from build123d import *

# Parameters (mm, degrees)
F1_DEPTH = 76.2
F0_R     = 3.17989
F2_DEPTH = 12.7
F0_R_2   = 3.190914
F3_DEPTH = 12.7
F0_W     = 38.1
F0_H     = 50.8
F4_DEPTH = 12.7


with BuildPart() as f1:
    # F0 (on Top) → F1 (new body)
    with BuildSketch(Plane.XY):
        Polygon((-63.963963, 7.02602), (-70.885196, 7.02602), (-70.885196, 6.905661), (-70.885196, -29.80398), (-20.085196, -29.80398), (-20.085196, 6.905661), (-20.085196, 7.02602), (-25.863963, 7.02602), align=None)
    extrude(amount=F1_DEPTH)

    # F0 (on Top) → F2 (join)
    with BuildSketch(Plane.XY):
        Polygon((-70.885196, -29.80398), (-70.885196, 6.905661), (-108.985196, 6.905661), (-108.985196, -29.924339), (-70.885196, -29.924339), align=None)
        with Locations((-89.978054, -11.557001)):
            Circle(F0_R, mode=Mode.SUBTRACT)
    extrude(amount=F2_DEPTH)

    # F0 (on Top) → F3 (join)
    with BuildSketch(Plane.XY):
        Polygon((-20.085196, 6.905661), (-20.085196, -29.80398), (-20.085196, -29.924339), (18.014804, -29.924339), (18.014804, 6.905661), align=None)
        with Locations((-0.353005, -11.161889)):
            Circle(F0_R_2, mode=Mode.SUBTRACT)
    extrude(amount=F3_DEPTH)

    # F0 (on Top) → F4 (join)
    with BuildSketch(Plane.XY):
        with Locations((-44.913963, 32.42602)):
            Rectangle(F0_W, F0_H)
        with Locations((-55.91448, 45.011953)):
            Circle(F0_R, mode=Mode.SUBTRACT)
        with Locations((-44.610804, 32.42602)):
            Circle(F0_R, mode=Mode.SUBTRACT)
        with Locations((-34.018744, 45.011953)):
            Circle(F0_R, mode=Mode.SUBTRACT)
    extrude(amount=F4_DEPTH)


solid = f1.part
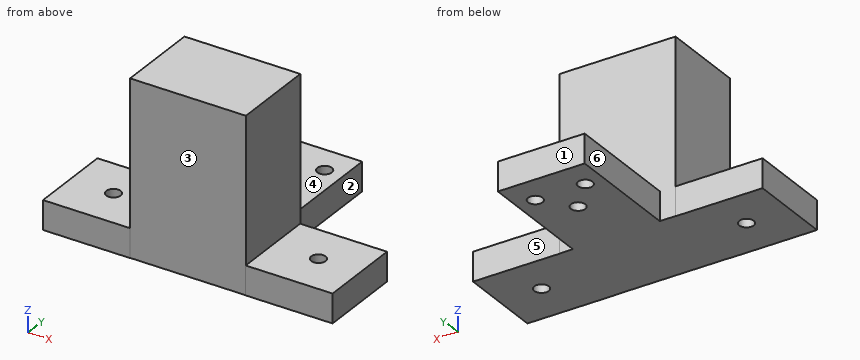
Geometry check sheet. Reference: the model listing, model coordinates, mm. Face numbers are marked on the shaded views. A direction names the side the tool comes from. Give positions to 0.01 mm unless a question says otherwise; leave off trailing zeros. Order: outer loops, then holes, each group sorted by start corner. A loop starts at its lowest first (then second) coordinate and runs counter-clockwise, first axis right, second up.
1) Material ranges on probe 1 along Z at (x, y) = (-1, 6); probe 2 along X at (y, z) = (-16.5, 29); probe 3 along Y at (x, z) = (-63.5, 60.5), recorded low to high.
Results are:
probe 1: z = 0 to 12.7
probe 2: x = -70.89 to -20.09
probe 3: y = -29.8 to 7.03
2) Cross-section at A-A (y = -6). Record the boundary of the cut face in (x, z), then the cut area to 3 significant figures.
Results are:
outline: (-108.99, 0) - (18.01, 0) - (18.01, 12.7) - (-20.09, 12.7) - (-20.09, 76.2) - (-70.89, 76.2) - (-70.89, 12.7) - (-108.99, 12.7) - close
area: 4,840 mm2
3) Gauge pin test, flat ends, axial feed: pin 1 (14 mm diameter, centred on x = 6, z = 9.5, fed in from +Y); pin 2 (10 mm diameter, centred on y = 36.5, z = 3.5, fed in from -X); pin 3 (11.5 mm diameter, centred on x = -40.5, y = 33, fed in from +Z). Record the tip position at first contact, or that the pin passes through.
Results are:
pin 1: stops at y = 6.91
pin 2: stops at x = -63.96
pin 3: stops at z = 12.7
4) Tool access check on the marked faces 4, 5 and 6. Record the directions out of +Z, -Z, +X, -X, +Y, -Y that give a thin tool (end or side, any length) a straight path to the whole face; none if there is none.
Results are:
face 4: +Z, +X, -X, +Y
face 5: +Z, -Z, +X, +Y
face 6: +Z, -Z, -X, +Y
5) Cross-section at C-C (x = -67.5). Record the boundary of the cut face in (y, z), then the cut area to 3 significant figures.
Results are:
outline: (-29.8, 0) - (7.03, 0) - (7.03, 76.2) - (-29.8, 76.2) - close
area: 2,810 mm2
6) Draft check along X on the marked faces 1, 2 and 3. Enter one of: released by +X, released by -X, zero draft, split by the parting line, or undercut.
Results are:
face 1: zero draft
face 2: released by +X
face 3: undercut
7) Cross-section at D-D (y = 14.5). Record the boundary of the cut face in (x, z).
Results are:
outline: (-63.96, 0) - (-25.86, 0) - (-25.86, 12.7) - (-63.96, 12.7) - close
8) Cross-section at B-B (z = 9.5). Record the boundary of the cut face in (x, y).
Results are:
outline: (-108.99, -29.92) - (-70.89, -29.92) - (-70.89, -29.8) - (-20.09, -29.8) - (-20.09, -29.92) - (18.01, -29.92) - (18.01, 6.91) - (-20.09, 6.91) - (-20.09, 7.03) - (-25.86, 7.03) - (-25.86, 57.83) - (-63.96, 57.83) - (-63.96, 7.03) - (-70.89, 7.03) - (-70.89, 6.91) - (-108.99, 6.91) - close; hole circle Ø6.36 at (-89.98, -11.56); hole circle Ø6.36 at (-55.91, 45.01); hole circle Ø6.36 at (-44.61, 32.43); hole circle Ø6.36 at (-34.02, 45.01); hole circle Ø6.38 at (-0.35, -11.16)
